Can you work these out from the drawing? Everything is in mm from the part's minimum corner. A direction names the side the tool comes from. Round coordinates to 2 decimals unless told otherwise and drop trailing zeros. Write each loop counter-clockwise with the first axis right and the second up, starting at its lowest first coordinate (ties: lowest second). Pieces come first, ordered by that corner, then holes. Notation, with made-up numbers: (-9.5, 21.5) - (49.5, 21.5) arc R19 ccw to (49.5, 37.5) - close; hole circle Ø9 at (26, 9.5). An arc over 180 degrees is marked (long way). One line per item, written item: value. Start each with the question number.
Item 1: If I drill on line 1 (Z direction, x = 16, y = 4); line 2 (Y direction, x = 37.5, z = 89) (3 decimals); line 3 (Y direction, x = 22, z = 88.55), over which ranges is the centre line in solid material (lowest first)?
Item 2: Thinking about a two-plate mould opening in X: for the marked faces 4, 5 and 6, which applies, released by +X, released by -X, zero draft, split by the parting line, or undercut?
Item 3: Imagine slicing it at B-B, the plane x = 6.5. Please give me the cut outline in (y, z) (3 decimals), then the cut area to 3 significant figures.
Item 4: Imagine slicing it at C-C, the plane y = 37.5. Please give me the cut outline in (x, z) (3 decimals).
Item 5: For the marked faces 1, 2 and 3, which set-ups out of +Z, -Z, +X, -X, +Y, -Y let a thin tool reach every point of the face, with its end or its side?
Item 6: Imagine slicing it at D-D, the plane x = 14. Please give me the cut outline in (y, z).
Item 7: Imagine slicing it at A-A, the plane y = 22. Please give me the cut outline in (x, z), then the cut area to 3 significant figures.
Item 8: For P1, Ø1.6, axis at x = 42.5, y = 14, coming from the -Z side; P2, Ø3, axis at x = 28.5, y = 35.5, coming from the -Z side; P3, Ø12, axis at x = 14, z = 22.5, coming from the +Y side; P4, Ø2.5, axis at x = 37.5, y = 6.5, coming from the -Z side, each with a flat end and sliding along its axis, tell me the tip position at first contact or that it passes through.
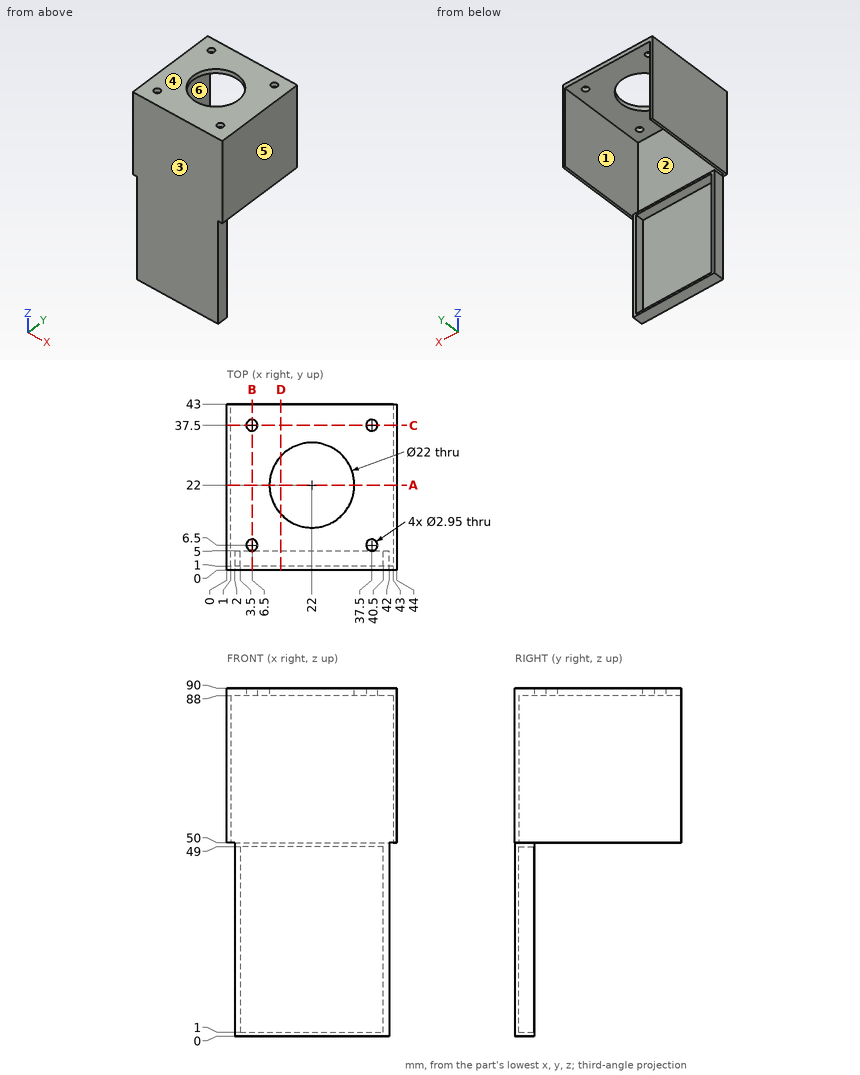
Values follow:
1. line 1: z = 0 to 1, 49 to 50, 88 to 90
1. line 2: y = 0 to 5.025, 7.975 to 36.025, 38.975 to 43
1. line 3: y = 0 to 11, 33 to 43
2. face 4: zero draft
2. face 5: released by +X
2. face 6: undercut
3. outline: (0, 0) - (5, 0) - (5, 1) - (1, 1) - (1, 49) - (5, 49) - (5, 50) - (1, 50) - (1, 88) - (5.025, 88) - (5.025, 90) - (0, 90) - close; (7.975, 88) - (36.025, 88) - (36.025, 90) - (7.975, 90) - close; (38.975, 88) - (43, 88) - (43, 90) - (38.975, 90) - close
3. area: 170 mm^2
4. outline: (0, 50) - (1, 50) - (1, 88) - (5.025, 88) - (5.025, 90) - (0, 90) - close; (7.975, 88) - (36.025, 88) - (36.025, 90) - (7.975, 90) - close; (38.975, 88) - (43, 88) - (43, 50) - (44, 50) - (44, 90) - (38.975, 90) - close
5. face 1: -Z, +Y
5. face 2: +Y
5. face 3: +Z, -Z, +X, -X, -Y
6. outline: (0, 0) - (5, 0) - (5, 1) - (1, 1) - (1, 49) - (5, 49) - (5, 50) - (1, 50) - (1, 88) - (14.45, 88) - (14.45, 90) - (0, 90) - close; (29.55, 88) - (43, 88) - (43, 90) - (29.55, 90) - close
7. outline: (0, 50) - (1, 50) - (1, 88) - (11, 88) - (11, 90) - (0, 90) - close; (33, 88) - (43, 88) - (43, 50) - (44, 50) - (44, 90) - (33, 90) - close
7. area: 120 mm^2
8. P1: stops at z = 50
8. P2: stops at z = 88
8. P3: stops at y = 1
8. P4: passes through
